Source: CAD feature listing. Evaluate the final solid. Frame: model axes, mm. A direction names the side the tool comes from. Give positions to 0.01 mm unless a question says otherwise; leave off trailing zeros. Loops run counter-clockwise (first coordinate to the right, second up) from the corner with the lowest first, then second, coordinate; pieces in that order, holes last. Notation, with made-up numbers: M -2.5,-28.5 L 22.5,-28.5 A12 cw 22.5,-23.5 Z; hole C 15,42.25 d2. An arc over 180 degrees is marked long. Answer in a Markdown table with one row per item.
```python
from build123d import *

# Parameters (mm, degrees)
EXTRUDE_1_DEPTH          = 18
SKETCH_2_R               = 17.875
SKETCH_2_R_2             = 1
EXTRUDE_2_DEPTH          = 18
PATTERN_CIRCULAR_3_COUNT = 12
SKETCH_3_R               = 1.1
CUT_EXTRUDE_1_DEPTH      = 19
PATTERN_CIRCULAR_4_COUNT = 4
SKETCH_4_R               = 2
CUT_EXTRUDE_2_DEPTH      = 10


with BuildPart() as part:
    # 草图1 → 凸台-拉伸1 (new body)
    with BuildSketch(Plane.XY):
        with BuildLine():
            ThreePointArc((3, 17.621453544), (0, 17.875), (-3, 17.621453544))
            ThreePointArc((-3, 17.621453544), (-2.381034791, 21.321544102), (-1, 24.809599575))
            ThreePointArc((-1, 24.809599575), (0, 24.830037117), (1, 24.809599575))
            ThreePointArc((1, 24.809599575), (2.381034791, 21.321544102), (3, 17.621453544))
        make_face()
    extrude_1 = extrude(amount=EXTRUDE_1_DEPTH)

    # 草图2 → 凸台-拉伸2 (add)
    with BuildSketch(Plane.XY):
        Circle(SKETCH_2_R)
        Circle(SKETCH_2_R_2, mode=Mode.SUBTRACT)
    extrude(amount=EXTRUDE_2_DEPTH)

    # 阵列(圆周)3: 凸台-拉伸1 ×12 about axis
    pattern_circular_3_axis = Axis((0, 0, 0), (0, 0, 1))
    for i in range(1, PATTERN_CIRCULAR_3_COUNT):
        add(extrude_1.rotate(pattern_circular_3_axis, i * 360 / PATTERN_CIRCULAR_3_COUNT))

    # 草图3 → 切除-拉伸1 (cut, through all)
    with BuildSketch(Plane(origin=(0, 0, 0), x_dir=(-1, 0, 0), z_dir=(0, 0, -1))):
        with Locations((0, 8)):
            Circle(SKETCH_3_R)
    cut_extrude_1 = extrude(amount=-CUT_EXTRUDE_1_DEPTH, mode=Mode.SUBTRACT)

    # 阵列(圆周)4: 切除-拉伸1 ×4 about axis
    pattern_circular_4_axis = Axis((0, 0, 0), (0, 0, 1))
    for i in range(1, PATTERN_CIRCULAR_4_COUNT):
        add(cut_extrude_1.rotate(pattern_circular_4_axis, i * 360 / PATTERN_CIRCULAR_4_COUNT), mode=Mode.SUBTRACT)

    # 草图4 → 切除-拉伸2 (cut)
    with BuildSketch(Plane.XY.offset(18)):
        with Locations((0, 8)):
            Circle(SKETCH_4_R)
        with Locations((8, 0)):
            Circle(SKETCH_4_R)
        with Locations((0, -8)):
            Circle(SKETCH_4_R)
        with Locations((-8, 0)):
            Circle(SKETCH_4_R)
    extrude(amount=-CUT_EXTRUDE_2_DEPTH, mode=Mode.SUBTRACT)


solid = part.part
```
Q1. Reachability of faces 1 (the cylindrical face through (0, -6, 13)), 2 (the cylindrical face through (21.271, 2.395, 8.874)), 3 (the cylindrical face through (-8.56, -19.62, 8.87)), 4 (the cylindrical face through (-17.26, 4.65, 8.87)) from +Z, -Z, +X, -X, +Y, -Y: full face, straight path, thin tool, end or side. Return the list, or none.
Values follow:
| item | result |
|---|---|
| face 1 | +Z |
| face 2 | +Z, -Z, +X |
| face 3 | +Z, -Z, -Y |
| face 4 | +Z, -Z, -X |
Q2. Ray query, probe 1 along Y at (x, z) = (0, 3.25); probe 2 along X at (y, z) = (-20, 15.5). Return the intervals inside material, ascending. Write a range as from..to.
Values follow:
| item | result |
|---|---|
| probe 1 | -24.83..-9.1, -6.9..-1, 1..6.9, 9.1..24.83 |
| probe 2 | -13.2..-8.96, -2.69..2.69, 8.96..13.2 |
Q3. Section query A-A (y = 0). Output: boundary loops of the cut face in (x, z).
Values follow:
| item | result |
|---|---|
| outline | M -24.83,0 L -9.1,0 L -9.1,8 L -10,8 L -10,18 L -24.83,18 Z; M -6.9,0 L -1,0 L -1,18 L -6,18 L -6,8 L -6.9,8 Z; M 1,0 L 6.9,0 L 6.9,8 L 6,8 L 6,18 L 1,18 Z; M 9.1,0 L 24.83,0 L 24.83,18 L 10,18 L 10,8 L 9.1,8 Z |
Q4. Contact query for flat-ended pins moving along their axis: pin 1 Ø6 at (x, z) = (-9.5, 2.5) entering from +Y; pin 2 Ø3.5 at (x, y) = (0, 8) entering from +Z; pin 3 Ø10 at (y, z) = (-9.5, 3) entering from -X. Output: stop coordinate, or through.
Values follow:
| item | result |
|---|---|
| pin 1 | y = 21.99 |
| pin 2 | z = 8 |
| pin 3 | x = -21.99 |
Q5. Section query D-D (z = 10.5). Give the number of separate pieces and of enclosed holes in the cut face, plus the area to 3 significant figures.
Values follow:
| item | result |
|---|---|
| separate pieces | 1 |
| enclosed holes | 5 |
| area | 1,330 mm^2 |
Q6. Mould query, pull axis Y, two halves, no side actions, for faces 5 (the cylindrical face through (4.65, 17.26, 8.87)), 6 (the cylindrical face through (-19.62, 8.56, 8.87)), 7 (the cylindrical face through (4.604, -17.272, 8.874)). Classes: +Y half, -Y half, draft (parallel to the pull), parting line (faces both ways), or undercut.
Values follow:
| item | result |
|---|---|
| face 5 | +Y half |
| face 6 | undercut |
| face 7 | -Y half |
Q7. Section query C-C (x = -19.5). Output: boundary loops of the cut face in (y, z), plus the area to 3 significant figures.
Values follow:
| item | result |
|---|---|
| outline | M -13.15,0 L -8.44,0 L -8.44,18 L -13.15,18 Z; M -2.79,0 L 2.79,0 L 2.79,18 L -2.79,18 Z; M 8.44,0 L 13.15,0 L 13.15,18 L 8.44,18 Z |
| area | 270 mm^2 |
